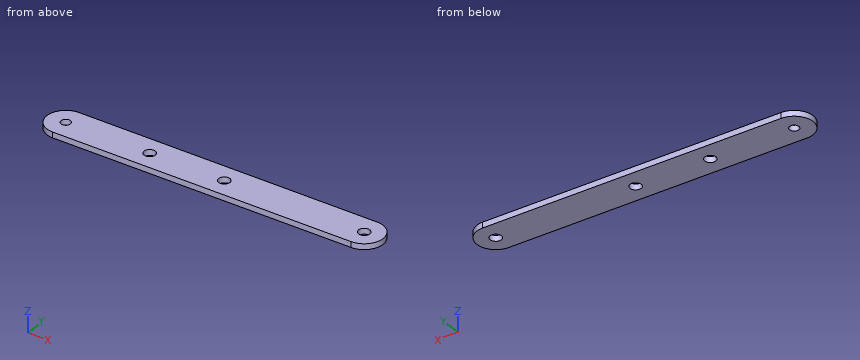
Autodesk Inventor part; units mm, degrees
ref_plane "YZ Plane" through (0, 0, 0) normal (1, 0, 0) x (0, 1, 0)
ref_plane "XZ Plane" through (0, 0, 0) normal (0, 1, 0) x (-1, 0, 0)
ref_plane "XY Plane" through (0, 0, 0) normal (0, 0, 1) x (1, 0, 0)
sketch "Szkic1" plane through (0, 0, 0) normal (0, 0, 1) x (1, 0, 0)
  line L0 (0, 0) -> (160, 0) construction
  line L1 (0, -10) -> (160, -10)
  line L2 (160, 10) -> (0, 10)
  arc A0 (0, 10) -> (0, -10) centre (0, 0) ccw
  arc A1 (160, -10) -> (160, 10) centre (160, 0) ccw
  point P0 (80, 0)
  point P1 (85, 0)
  point P2 (45, 0)
  dimension "d0" = 160
  dimension "d1" = 20
  dimension "d2" = 75
  dimension "d12" = 45
extrude "Wyciągnięcie proste1" add sketch "Szkic1" along normal blind 3
hole "Otwór1" at (160, 0, 0) at (85, 0, 0) at (45, 0, 0) direction (0, 0, 1) diameter 6 end through all
hole "Otwór2" at (0, 0, 0) direction (0, 0, 1) diameter 5 end through all
properties part number "glowny_wahacz"
For this review, take the finished solid that the model builds, in its own axes (mm). Give positions to 0.01 mm unless a question says otherwise; leave off trailing zeros. Write each loop counter-clockwise with the first axis right and the second up, starting at its lowest first coordinate (ties: lowest second). Pieces come first, ordered by that corner, then holes.
Item 1: Take a section at B-B (y = 0). Give the boundary of the cut face in (x, z).
Item 2: Take a section at C-C (x = 85). Give the boundary of the cut face in (y, z), and give its area (3 significant figures).
Item 3: Insertion check: P1, Ø3.5, axis at x = 160, y = 0, coming from the -Z side. The pin has a flat end and moves straight along its axis. Give the tip position at first contact, or say it passes through.
Item 4: Take a section at A-A (z = 2.45). Give the boundary of the cut face in (x, y).
Item 5: Wall thickness on probe 1 along X at (y, z) = (0, 2.25); probe 2 along X at (y, z) = (1.75, 0.45); probe 3 along Y at (x, z) = (0, 0.9): over which ranges is each line inside the solid? List them lowest first.
Item 6: Take a section at D-D (y = 6.75). Give the boundary of the cut face in (x, z).
Established:
1. outline: (-10, 0) - (-2.5, 0) - (-2.5, 3) - (-10, 3) - close; (2.5, 0) - (42, 0) - (42, 3) - (2.5, 3) - close; (48, 0) - (82, 0) - (82, 3) - (48, 3) - close; (88, 0) - (157, 0) - (157, 3) - (88, 3) - close; (163, 0) - (170, 0) - (170, 3) - (163, 3) - close
2. outline: (-10, 0) - (-3, 0) - (-3, 3) - (-10, 3) - close; (3, 0) - (10, 0) - (10, 3) - (3, 3) - close
2. area: 42.0 mm2
3. P1: passes through
4. outline: (0, -10) - (160, -10) arc R10 ccw to (160, 10) - (0, 10) arc R10 ccw to start; hole circle Ø5 at (0, 0); hole circle Ø6 at (45, 0); hole circle Ø6 at (85, 0); hole circle Ø6 at (160, 0)
5. probe 1: x = -10 to -2.5, 2.5 to 42, 48 to 82, 88 to 157, 163 to 170
5. probe 2: x = -9.85 to -1.79, 1.79 to 42.56, 47.44 to 82.56, 87.44 to 157.56, 162.44 to 169.85
5. probe 3: y = -10 to -2.5, 2.5 to 10
6. outline: (-7.38, 0) - (167.38, 0) - (167.38, 3) - (-7.38, 3) - close
